Could you check a few things on this model? Use its own coordinates, in mm. Face numbers are marked on the shaded views. A direction names the side the tool comes from. Give positions to 0.01 mm unless a question says otherwise; leave off trailing zeros. Loops run counter-clockwise (first coordinate to the right, second up) from the corner with the lowest first, then second, coordinate; pieces in that order, holes last. Notation, with made-up numbers: (67.25, 2) -> (90.25, 2) arc R21 ccw to (90.25, 41) -> close; hole circle Ø5 at (26, 72). An arc over 180 degrees is marked (long way). Put each result on its own line as item: value.
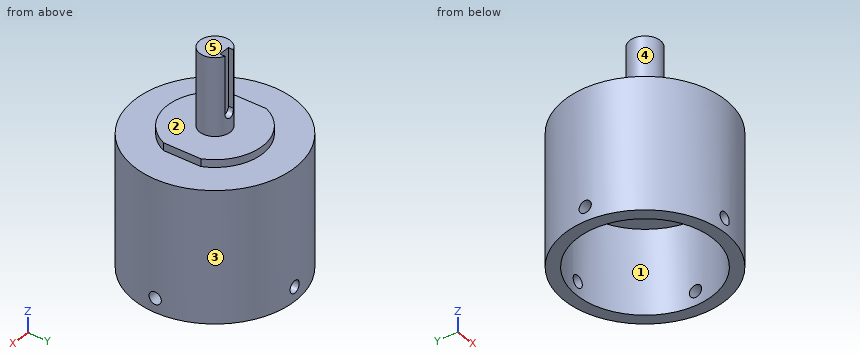
```python
from build123d import *

# Parameters (mm, degrees)
SKETCH_1_R               = 21
SKETCH_1_R_2             = 17.75
EXTRUDE_1_DEPTH          = 34.2
EXTRUDE_START            = -12.2
SKETCH_2_R               = 21
EXTRUDE_2_DEPTH          = 12.2
EXTRUDE_3_DEPTH          = 2
SKETCH_4_R               = 4
EXTRUDE_4_DEPTH          = 20.2
SKETCH_5_R               = 1.6
CUT_EXTRUDE_1_DEPTH      = 64.741352355
PATTERN_CIRCULAR_1_COUNT = 4
CUT_EXTRUDE_2_DEPTH      = 1.6


with BuildPart() as part:
    # ｽｹｯﾁ1 → ﾎﾞｽ - 押し出し1 (new body)
    with BuildSketch(Plane.XY):
        Circle(SKETCH_1_R)
        Circle(SKETCH_1_R_2, mode=Mode.SUBTRACT)
    extrude(amount=EXTRUDE_1_DEPTH)

    # ｽｹｯﾁ2 → ﾎﾞｽ - 押し出し2 (add)
    with BuildSketch(Plane.XY.offset(34.2).offset(EXTRUDE_START)):
        Circle(SKETCH_2_R)
    extrude(amount=EXTRUDE_2_DEPTH)

    # ｽｹｯﾁ3 → ﾎﾞｽ - 押し出し3 (add)
    with BuildSketch(Plane.XY.offset(34.2)):
        with BuildLine():
            Line((-11.5, -4.898979486), (-11.5, 4.898979486))
            ThreePointArc((-11.5, 4.898979486), (0, 12.5), (11.5, 4.898979486))
            Line((11.5, 4.898979486), (11.5, -4.898979486))
            ThreePointArc((11.5, -4.898979486), (0, -12.5), (-11.5, -4.898979486))
        make_face()
    extrude(amount=EXTRUDE_3_DEPTH)

    # ｽｹｯﾁ4 → ﾎﾞｽ - 押し出し4 (add)
    with BuildSketch(Plane.XY.offset(36.2)):
        Circle(SKETCH_4_R)
    extrude(amount=EXTRUDE_4_DEPTH)

    # ｽｹｯﾁ5 → ｶｯﾄ - 押し出し1 (cut, through all)
    with BuildSketch(Plane(origin=(0, 0, 0), x_dir=(1, 0, 0), z_dir=(0, 1, 0))):
        with Locations(Location((0, -3.7, 0), (0, 0, 270))):
            Circle(SKETCH_5_R)
    cut_extrude_1 = extrude(amount=-CUT_EXTRUDE_1_DEPTH, mode=Mode.SUBTRACT)

    # 円形ﾊﾟﾀｰﾝ1: ｶｯﾄ - 押し出し1 ×4 about axis
    pattern_circular_1_axis = Axis((0, 0, 34.2), (0, 0, -1))
    for i in range(1, PATTERN_CIRCULAR_1_COUNT):
        add(cut_extrude_1.rotate(pattern_circular_1_axis, i * 360 / PATTERN_CIRCULAR_1_COUNT), mode=Mode.SUBTRACT)

    # ｽｹｯﾁ7 → ｶｯﾄ - 押し出し2 (cut)
    with BuildSketch(Plane(origin=(0, 4, 0), x_dir=(1, 0, 0), z_dir=(0, 1, 0))):
        with BuildLine():
            Line((-1.5, -56.4), (-1.5, -41.4))
            ThreePointArc((-1.5, -41.4), (0, -39.9), (1.5, -41.4))
            Line((1.5, -41.4), (1.5, -56.4))
            ThreePointArc((1.5, -56.4), (0, -57.9), (-1.5, -56.4))
        make_face()
    extrude(amount=-CUT_EXTRUDE_2_DEPTH, mode=Mode.SUBTRACT)


solid = part.part
```
1. I need wall thicknesses on line 1 (Z direction, x = 0, y = -20); line 2 (X direction, y = 0, z = 17); line 3 (Z direction, x = -2.5, y = 14). Which ranges of each line are inside material? Lowest first, please.
Recorded:
line 1: z = 0 to 2.1, 5.3 to 34.2
line 2: x = -21 to -17.75, 17.75 to 21
line 3: z = 22 to 34.2
2. If we section it at C-C (z = 3.7): List the corners of the cut face in (x, y) for me, then the cut area to 3 significant figures.
Recorded:
outline: (-20.94, -1.6) arc R21 ccw to (-1.6, -20.94) -> (-1.6, -17.68) arc R17.75 cw to (-17.68, -1.6) -> close; (-20.94, 1.6) -> (-17.68, 1.6) arc R17.75 cw to (-1.6, 17.68) -> (-1.6, 20.94) arc R21 ccw to start; (1.6, -20.94) arc R21 ccw to (20.94, -1.6) -> (17.68, -1.6) arc R17.75 cw to (1.6, -17.68) -> close; (1.6, 17.68) arc R17.75 cw to (17.68, 1.6) -> (20.94, 1.6) arc R21 ccw to (1.6, 20.94) -> close
area: 354 mm^2
3. Thinking about a two-plate mould opening in Y: for the marked faces 1, 2 and 3, which applies, pulls with the +Y half, pulls with the -Y half, needs draft (parallel to the pull), parting line crosses it, or undercut?
Recorded:
face 1: undercut
face 2: needs draft
face 3: parting line crosses it
4. If we section it at A-A (y = 0): List the corners of the cut face in (x, z) for me.
Recorded:
outline: (-21, 0) -> (-17.75, 0) -> (-17.75, 2.1) -> (-21, 2.1) -> close; (-21, 5.3) -> (-17.75, 5.3) -> (-17.75, 22) -> (17.75, 22) -> (17.75, 5.3) -> (21, 5.3) -> (21, 34.2) -> (11.5, 34.2) -> (11.5, 36.2) -> (4, 36.2) -> (4, 56.4) -> (-4, 56.4) -> (-4, 36.2) -> (-11.5, 36.2) -> (-11.5, 34.2) -> (-21, 34.2) -> close; (17.75, 0) -> (21, 0) -> (21, 2.1) -> (17.75, 2.1) -> close
5. I'm going to push flat-ended pins straight in: pin 1 (0.7 mm diameter, centred on y = 3, z = 52.5, fed in from -X); pin 2 (10 mm diameter, centred on x = 16, y = -5.5, fed in from +Z); pin 3 (3 mm diameter, centred on y = 7, z = 16, fed in from -X). Where does each tip first touch, or does it pass through?
Recorded:
pin 1: stops at x = -3
pin 2: stops at z = 36.2
pin 3: stops at x = -20.27
6. For the marked faces 4 and 5, which set-ups out of +Z, -Z, +X, -X, +Y, -Y let a thin tool reach every point of the face, with its end or its side?
Recorded:
face 4: +Z
face 5: +Z, +X, -X, +Y, -Y
7. If we section it at B-B (x = 0): List the corners of the cut face in (y, z) for me, then the cut area to 3 significant figures.
Recorded:
outline: (-21, 0) -> (-17.75, 0) -> (-17.75, 2.1) -> (-21, 2.1) -> close; (-21, 5.3) -> (-17.75, 5.3) -> (-17.75, 22) -> (17.75, 22) -> (17.75, 5.3) -> (21, 5.3) -> (21, 34.2) -> (12.5, 34.2) -> (12.5, 36.2) -> (4, 36.2) -> (4, 39.9) -> (2.4, 39.9) -> (2.4, 56.4) -> (-4, 56.4) -> (-4, 36.2) -> (-12.5, 36.2) -> (-12.5, 34.2) -> (-21, 34.2) -> close; (17.75, 0) -> (21, 0) -> (21, 2.1) -> (17.75, 2.1) -> close
area: 820 mm^2
8. If we section it at D-D (z = 13.5): List the corners of the cut face in (x, y) for me, then the cut area to 3 significant figures.
Recorded:
outline: circle Ø42 at (0, 0); hole circle Ø35.5 at (0, 0)
area: 396 mm^2
